```python
from build123d import *

# Parameters (mm, degrees)
BOSS_EXTRUDE1_DEPTH = 2.54
FILLET1_R           = 0.254
CUT_EXTRUDE1_DEPTH  = 2.54


with BuildPart() as part:
    # Sketch1 → Boss-Extrude1 (new body)
    with BuildSketch(Plane(origin=(0, 0, 0), x_dir=(0, 0, -1), z_dir=(1, 0, 0))):
        with BuildLine():
            ThreePointArc((6.35, 0), (0, -6.35), (-6.35, 0))
            Line((-6.35, 0), (-6.35, -43.036593364))
            Line((-6.35, -43.036593364), (6.35, -43.036593364))
            Line((6.35, -43.036593364), (6.35, 0))
        make_face()
    extrude(amount=BOSS_EXTRUDE1_DEPTH)

    # Fillet1
    fillet1_edges = [part.edges().sort_by_distance(p)[0] for p in [
        (1.27, 0, -6.35),
        (1.27, 0, 6.35),
    ]]
    fillet(fillet1_edges, radius=FILLET1_R)

    # Sketch2 → Cut-Extrude1 (cut)
    with BuildSketch(Plane.ZY):
        with BuildLine():
            Line((1.984375, -14.393108905), (1.984375, -37.585187193))
            ThreePointArc((1.984375, -37.585187193), (0, -39.569562193), (-1.984375, -37.585187193))
            Line((-1.984375, -37.585187193), (-1.984375, -14.393108905))
            ThreePointArc((-1.984375, -14.393108905), (0, -12.408733905), (1.984375, -14.393108905))
        make_face()
    extrude(amount=-CUT_EXTRUDE1_DEPTH, mode=Mode.SUBTRACT)


solid = part.part
```
Here's how the part is built. I have some questions about the finished solid (model axes, mm). A direction names the side the tool comes from. Coordinates: 2 decimals unless noted, no trailing zeros. Loops run counter-clockwise (first coordinate to the right, second up) from the corner with the lowest first, then second, coordinate; pieces in that order, holes last. Notation, with made-up numbers: (-9.5, 85) - (8.5, 85) arc R10 ccw to (8.5, 94) - close; hole circle Ø3 at (-35, -32.5). An arc over 180 degrees is marked (long way). Return JSON: item names as keys, results as strings. Group by question number.
Item 1: If we section it at D-D on z = -4.75: Write out the boundary of the cut face in (x, y).
Item 2: I need wall thicknesses on line 1 (Z direction, x = 0.3, y = -33); line 2 (Y direction, x = 0.8, z = 0); line 3 (Z direction, x = 0.35, y = -38). Which ranges of each line are inside material? Lowest first, please. Write a range as from..to.
Item 3: If we section it at B-B on y = -33: Write out the boundary of the cut face in (x, z), and give its area (3 significant figures).
Item 4: If we section it at A-A on z = 0: Write out the boundary of the cut face in (x, y).
Item 5: We'd pull the mould along Y, two halves only. Please class faces 1 (the face through (1, -23, 6.35)), 2 (the face through (1.25, -6.35, -0.1)), 3 (the face through (1.25, -12.41, -0.04)), 4 (the face through (1, -26, -1.984)): +Y half, -Y half, draft (parallel to the pull), parting line (faces both ways), or undercut.
Item 6: If we section it at C-C on z = 2.5: Write out the boundary of the cut face in (x, y).
Item 7: On a 3-axis mill with a long thin cutter (end or side, diameter ignored), from which of +Z, -Z, +X, -X, +Y, -Y can I reach the whole of each face in a straight line? I mean faces 5 (the face through (1.25, -39.57, 0.04)), 6 (the face through (1, -43.037, 0)). Say none if no direction works.
Calculated:
{
 "1": {"outline": "(0, -43.04) - (2.54, -43.04) - (2.54, -4.21) - (0, -4.21) - close"},
 "2": {"line 1": "z = -6.35..-1.98, 1.98..6.35", "line 2": "y = -43.04..-39.57, -12.41..-6.35", "line 3": "z = -6.35..-1.94, 1.94..6.35"},
 "3": {"outline": "(0, -6.35) - (2.54, -6.35) - (2.54, -1.98) - (0, -1.98) - close; (0, 1.98) - (2.54, 1.98) - (2.54, 6.35) - (0, 6.35) - close", "area": "22.2 mm^2"},
 "4": {"outline": "(0, -43.04) - (2.54, -43.04) - (2.54, -39.57) - (0, -39.57) - close; (0, -12.41) - (2.54, -12.41) - (2.54, -6.35) - (0, -6.35) - close"},
 "5": {"face 1": "draft", "face 2": "+Y half", "face 3": "undercut", "face 4": "undercut"},
 "6": {"outline": "(0, -43.04) - (2.54, -43.04) - (2.54, -5.84) - (0, -5.84) - close"},
 "7": {"face 5": "+X, -X", "face 6": "+Z, -Z, +X, -X, -Y"}
}
